Design review of the part built by this model. Coordinates are the model's own, in mm. Face numbers are marked on the shaded views. Give positions to 0.01 mm unless a question says otherwise; leave off trailing zeros. Loops run counter-clockwise (first coordinate to the right, second up) from the corner with the lowest first, then second, coordinate; pieces in that order, holes last. Notation, with made-up numbers: (25.5, 45) -> (68.5, 45) arc R21 cw to (68.5, 49) -> close; hole circle Ø11 at (71.5, 74). An arc over 180 degrees is marked (long way). Answer in a Markdown table with one row per item. Add a question column.
(1) For line 1 (X direction, y = -6.75, z = 11.75); line 2 (Y direction, x = -3, z = 4.25); line 3 (X direction, y = 1.75, z = 4), list the stretches that pass through material, from the lowest coordinate up.
(2) For pin 1 (5 mm diameter, centred on x = 6.5, y = 8.5, fed in from +Z); pin 2 (3 mm diameter, centred on y = 7, z = 6, fed in from -X); pin 3 (8 mm diameter, centred on y = -9, z = 12, fed in from +X); pin 4 (1.5 mm diameter, centred on y = -9.5, z = 13, fed in from -X), all flat-tipped, find the tip position at first contact; note any pin that passes through.
(3) Consider section A-A on z = 9.5. Write out the cut boundary in (x, y).
(4) Consider section B-B on y = 0. Write out the cut boundary in (x, z), then the cut area to 3 significant figures.
(5) Consider section C-C on x = 0. Write out the cut boundary in (y, z).
(6) Consider section D-D on z = 2. Write out the cut boundary in (x, y), then the cut area to 3 significant figures.
(7) Draft analysis for pull direction X (two halves, no side actions). For the marked faces 1, 2 and 3, state which applies: +X half, -X half, draft (parallel to the pull), parting line (faces both ways), or undercut.
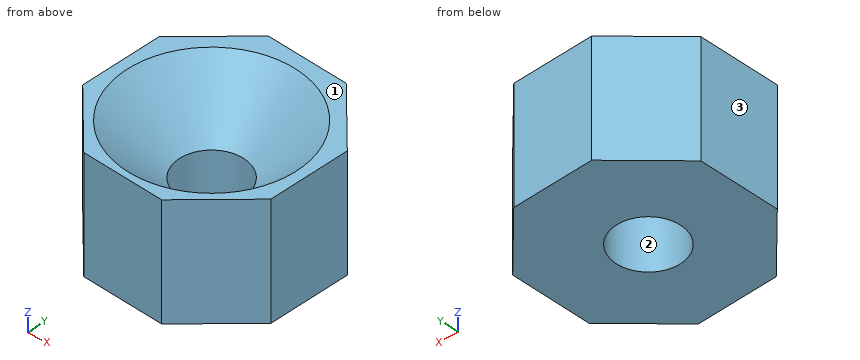
from build123d import *

# Parameters (mm, degrees)
F1_DEPTH       = 15
F3_D           = 8.5
F3_CSINK_D     = 22.4
F3_CSINK_ANGLE = 90


with BuildPart() as f1:
    # F0 (on Top) → F1 (new body)
    with BuildSketch(Plane.XY):
        Polygon((12.2918519161, -5.1738469947), (12.6896912522, 5.1738469947), (5.654081555, 12.7720864765), (-4.6936124343, 13.1699258125), (-12.2918519161, 6.1343161154), (-12.6896912522, -4.2133778739), (-5.654081555, -11.8116173557), (4.6936124343, -12.2094566918), align=None)
    extrude(amount=F1_DEPTH)

    # F3 (through all)
    with Locations(Plane.XY.offset(15)):
        with Locations((0, 0)):
            CounterSinkHole(F3_D / 2, F3_CSINK_D / 2, counter_sink_angle=F3_CSINK_ANGLE)


solid = f1.part
Values follow:
| question | item | result |
|---|---|---|
| 1 | line 1 | -10.34 to -4.2, 4.2 to 10.59 |
| 1 | line 2 | -11.91 to -3.01, 3.01 to 13.1 |
| 1 | line 3 | -12.46 to -3.87, 3.87 to 12.56 |
| 2 | pin 1 | z = 15 |
| 2 | pin 2 | x = -12.32 |
| 2 | pin 3 | x = 12.3 |
| 2 | pin 4 | x = -8.49 |
| 3 | outline | (-12.69, -4.21) -> (-5.65, -11.81) -> (4.69, -12.21) -> (12.29, -5.17) -> (12.69, 5.17) -> (5.65, 12.77) -> (-4.69, 13.17) -> (-12.29, 6.13) -> close; hole circle Ø11.4 at (0, 0) |
| 4 | outline | (-12.53, 0) -> (-4.25, 0) -> (-4.25, 8.05) -> (-11.2, 15) -> (-12.53, 15) -> close; (4.25, 0) -> (12.49, 0) -> (12.49, 15) -> (11.2, 15) -> (4.25, 8.05) -> close |
| 4 | area | 199 mm2 |
| 5 | outline | (-12.03, 0) -> (-4.25, 0) -> (-4.25, 8.05) -> (-11.2, 15) -> (-12.03, 15) -> close; (4.25, 0) -> (12.99, 0) -> (12.99, 15) -> (11.2, 15) -> (4.25, 8.05) -> close |
| 6 | outline | (-12.69, -4.21) -> (-5.65, -11.81) -> (4.69, -12.21) -> (12.29, -5.17) -> (12.69, 5.17) -> (5.65, 12.77) -> (-4.69, 13.17) -> (-12.29, 6.13) -> close; hole circle Ø8.5 at (0, 0) |
| 6 | area | 461 mm2 |
| 7 | face 1 | draft |
| 7 | face 2 | undercut |
| 7 | face 3 | -X half |
